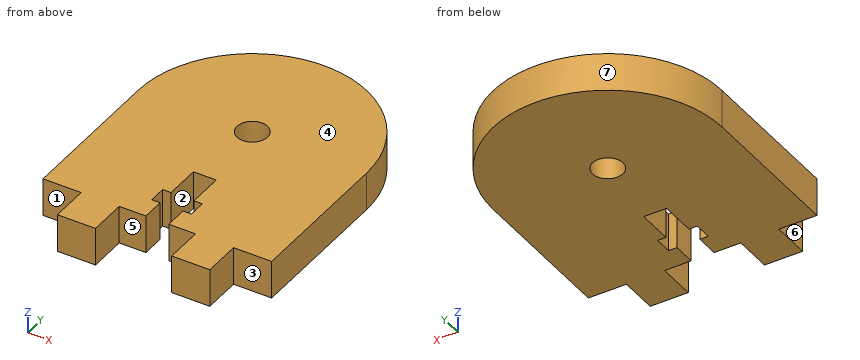
from build123d import *

# Parameters (mm, degrees)
SKETCH1_R           = 2
BOSS_EXTRUDE1_DEPTH = 5


with BuildPart() as part:
    # Sketch1 → Boss-Extrude1 (new body)
    with BuildSketch(Plane.XY):
        with BuildLine():
            Line((-10, 0), (-15, 0))
            Line((-15, 0), (-15, 20))
            ThreePointArc((-15, 20), (0, 35), (15, 20))
            Line((15, 20), (15, 0))
            Line((15, 0), (10, 0))
            Line((10, 0), (10, -5))
            Line((10, -5), (5, -5))
            Line((5, -5), (5, 0))
            Line((5, 0), (1.5, 0))
            Line((1.5, 0), (1.5, 3))
            Line((1.5, 3), (2.6, 3))
            Line((2.6, 3), (2.6, 5.3))
            Line((2.6, 5.3), (1.5, 5.3))
            Line((1.5, 5.3), (1.5, 10))
            Line((1.5, 10), (-1.5, 10))
            Line((-1.5, 10), (-1.5, 5.3))
            Line((-1.5, 5.3), (-2.6, 5.3))
            Line((-2.6, 5.3), (-2.6, 3))
            Line((-2.6, 3), (-1.5, 3))
            Line((-1.5, 3), (-1.5, 0))
            Line((-1.5, 0), (-5, 0))
            Line((-5, 0), (-5, -5))
            Line((-5, -5), (-10, -5))
            Line((-10, -5), (-10, 0))
        make_face()
        with Locations((0, 20)):
            Circle(SKETCH1_R, mode=Mode.SUBTRACT)
    extrude(amount=BOSS_EXTRUDE1_DEPTH)


solid = part.part
Check sheet for the modelled part. Datum: model origin and axes. Units: mm. Face numbers are marked on the shaded views. A direction names the side the tool comes from. Round coordinates to 2 decimals unless told otherwise and drop trailing zeros. Write each loop counter-clockwise with the first axis right and the second up, starting at its lowest first coordinate (ties: lowest second). Pieces come first, ordered by that corner, then holes. Notation, with made-up numbers: (49.5, 51.25) -> (96.5, 51.25) arc R14 ccw to (96.5, 63.25) -> close; hole circle Ø6 at (39, 55.25). An arc over 180 degrees is marked (long way). Answer as CSV lines item,"result". Start each with the question number.
1) Section check D-D on y = 29. Enter the section's corners in (x, z).
2) Release check for a two-part mould opening along X. For the marked faces 4, 5, 6 and 7 record: pulls with the +X half, pulls with the -X half, needs draft (parallel to the pull), parting line crosses it, or undercut.
3) Section check A-A on x = 0. Enter the section's corners in (y, z).
4) Go/stop test with flat-tipped pins: P1, Ø1.2, axis at x = -2.5, z = 2, coming from the +Y side; P2, Ø1, axis at x = -2.5, z = 3, coming from the -Y side; P3, Ø1.5, axis at y = -3, z = 2.5, coming from the -X side. Record where each tip stops, or that it passes through.
5) Section check B-B on y = -0.5. Enter the section's corners in (x, z).
6) Section check C-C on z = 1.75. Enter the section's corners in (x, y).
7) Material ranges on line 1 (Y direction, x = 0, z = 1.55); line 2 (X direction, y = -1, z = 4.85); line 3 (X direction, y = 5, z = 4.35), recorded low to high. Write a range as from..to.
8) Tool access check on the marked faces 1, 2 and 3. Record the directions out of +Z, -Z, +X, -X, +Y, -Y that give a thin tool (end or side, any length) a straight path to the whole face; none if there is none.
Found:
1,outline,"(-12, 0) -> (12, 0) -> (12, 5) -> (-12, 5) -> close"
2,face 4,"needs draft"
2,face 5,"undercut"
2,face 6,"pulls with the -X half"
2,face 7,"parting line crosses it"
3,outline,"(10, 0) -> (18, 0) -> (18, 5) -> (10, 5) -> close; (22, 0) -> (35, 0) -> (35, 5) -> (22, 5) -> close"
4,P1,"stops at y = 34.88"
4,P2,"stops at y = 0"
4,P3,"stops at x = -10"
5,outline,"(-10, 0) -> (-5, 0) -> (-5, 5) -> (-10, 5) -> close; (5, 0) -> (10, 0) -> (10, 5) -> (5, 5) -> close"
6,outline,"(-15, 0) -> (-10, 0) -> (-10, -5) -> (-5, -5) -> (-5, 0) -> (-1.5, 0) -> (-1.5, 3) -> (-2.6, 3) -> (-2.6, 5.3) -> (-1.5, 5.3) -> (-1.5, 10) -> (1.5, 10) -> (1.5, 5.3) -> (2.6, 5.3) -> (2.6, 3) -> (1.5, 3) -> (1.5, 0) -> (5, 0) -> (5, -5) -> (10, -5) -> (10, 0) -> (15, 0) -> (15, 20) arc R15 ccw to (-15, 20) -> close; hole circle Ø4 at (0, 20)"
7,line 1,"y = 10..18, 22..35"
7,line 2,"x = -10..-5, 5..10"
7,line 3,"x = -15..-2.6, 2.6..15"
8,face 1,"+Z, -Z, -X, -Y"
8,face 2,"+Z, -Z, -Y"
8,face 3,"+Z, -Z, +X, -Y"
